Input: dimensioned drawing with shaded views. Units: mm. Origin: part minimum x, y, z. Round coordinates to 2 decimals unless told otherwise and drop trailing zeros. Order: outer loops, then holes, each group sorted by start corner. A loop starts at its lowest first (then second) coordinate and runs counter-clockwise, first axis right, second up. Notation, with made-up numbers: (-36, 79) - (-7, 79) arc R20 ccw to (-7, 111) - close; hole circle Ø5 at (70.5, -8). An arc over 180 degrees is marked (long way). Return JSON: item names as keys, results as strings. Group by question number.
1) Ray query, line 1 (Z direction, x = 3.6, y = 1.7); line 2 (Y direction, x = 5.5, z = 1). Return the intervals inside material, ascending. Write a range as from..to.
2) Section B-B, the plane z = 2.75. Return loops of the section in (x, y).
3) Section C-C, the plane y = 3.35. Return loops of the section in (x, z).
4) Section D-D, the plane x = 1. Return loops of the section in (y, z).
5) Contact query for a flat-ended pin moving along its axis: P1, Ø2, axis at x = 4, z = 3.5, coming from the -Y side. Output: stop coordinate, or through.
6) Mould query, pull axis X, two halves, no side actions, for the marked faces 1, 2 and 3. Classes: pulls with the +X half, pulls with the -X half, needs draft (parallel to the pull), parting line crosses it, or undercut.
7) Section A-A, the plane x = 3.6. Return loops of the section in (y, z).
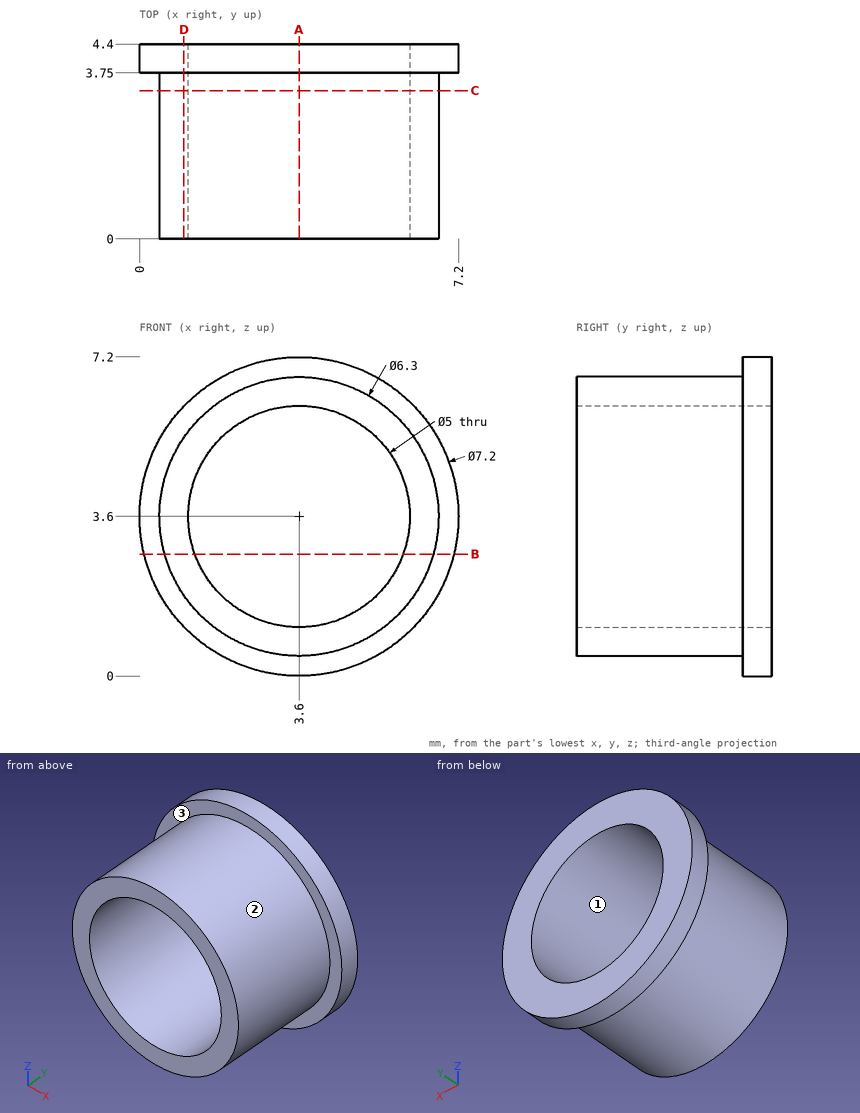
Geometry check:
{
 "1": {"line 1": "0.45..1.1, 6.1..6.75", "line 2": "3.75..4.4"},
 "2": {"outline": "(0.1, 3.75) - (0.57, 3.75) - (0.57, 0) - (1.25, 0) - (1.25, 4.4) - (0.1, 4.4) - close; (5.95, 0) - (6.63, 0) - (6.63, 3.75) - (7.1, 3.75) - (7.1, 4.4) - (5.95, 4.4) - close"},
 "3": {"outline": "circle Ø6.3 at (3.6, 3.6); hole circle Ø5 at (3.6, 3.6)"},
 "4": {"outline": "(0, 1.82) - (3.75, 1.82) - (3.75, 1.11) - (4.4, 1.11) - (4.4, 6.09) - (3.75, 6.09) - (3.75, 5.38) - (0, 5.38) - close"},
 "5": {"P1": "through"},
 "6": {"face 1": "undercut", "face 2": "parting line crosses it", "face 3": "needs draft"},
 "7": {"outline": "(0, 0.45) - (3.75, 0.45) - (3.75, 0) - (4.4, 0) - (4.4, 1.1) - (0, 1.1) - close; (0, 6.1) - (4.4, 6.1) - (4.4, 7.2) - (3.75, 7.2) - (3.75, 6.75) - (0, 6.75) - close"}
}
